from build123d import *

# Parameters (mm, degrees)
F0_W        = 186.2502396107
F0_H        = 130.5641233921
F1_DEPTH    = 50
F2_R        = 33.843412588
F3_DEPTH    = 153
F5_DEPTH    = 98
F6_T        = -2.5
F7_DEPTH    = 34.7
F8_T1_DEPTH = 77.2897189396
F8_T3_DEPTH = 80.4969668156
F8_T5_DEPTH = 71.5460241694


# Not quite as in the source:
# - a fillet or chamfer that OpenCascade refuses, or shapes differently, is made with other operations: its cross-section is extruded or revolved along the edge and cut away or added


with BuildPart() as f1:
    # F0 (on Top) → F1 (new body)
    with BuildSketch(Plane.XY):
        with Locations((-4.4038519263, -2.9969513416)):
            Rectangle(F0_W, F0_H)
    extrude(amount=F1_DEPTH)

    # F2 (on face) → F3 (cut)
    with BuildSketch(Plane(origin=(0, 0, 0), x_dir=(1, 0, 0), z_dir=(0, 0, -1))):
        with Locations((-44.7623804212, 0)):
            Circle(F2_R)
    extrude(amount=-F3_DEPTH, mode=Mode.SUBTRACT)

    # F4 (on face) → F5 (cut)
    with BuildSketch(Plane.XY.offset(50)):
        with BuildLine():
            Line((88.721267879, 62.2851103544), (43.5578748584, 62.2851103544))
            ThreePointArc((43.5578748584, 62.2851103544), (52.9449353899, 20.5157751148), (88.721267879, -2.9969513416))
            Line((88.721267879, -2.9969513416), (88.721267879, 62.2851103544))
        make_face()
    extrude(amount=-F5_DEPTH, mode=Mode.SUBTRACT)

    # F6
    f6_openings = [f1.faces().sort_by_distance(p)[0] for p in [
        (-26.985548, 62.28511, 25),
    ]]
    offset(amount=F6_T, openings=f6_openings)

    # F7 (add): a face of the model
    f7_faces = [f1.faces().sort_by_distance(p)[0] for p in [
        (-5.8734353471, -8.457374128, 50),
    ]]
    extrude(f7_faces, amount=-F7_DEPTH)

    # F8: fillet of radius 5.4579437879 on 5 edges, made by hand

    # F8_s2 → F8_t1 (cut)
    with BuildSketch(Plane.XY.offset(-13.6448594698)):
        with BuildLine():
            ThreePointArc((-97.5289717317, -62.8210692498), (-95.9303770075, -66.6804183135), (-92.0710279438, -68.2790130377))
            Line((-92.0710279438, -68.2790130377), (-97.5289717317, -68.2790130377))
            Line((-97.5289717317, -68.2790130377), (-97.5289717317, -62.8210692498))
        make_face()
        with BuildLine():
            ThreePointArc((83.2633240911, -68.2790130377), (87.1226731549, -66.6804183135), (88.721267879, -62.8210692498))
            Line((88.721267879, -62.8210692498), (88.721267879, -68.2790130377))
            Line((88.721267879, -68.2790130377), (83.2633240911, -68.2790130377))
        make_face()
        with BuildLine():
            ThreePointArc((-92.0710279438, 62.2851103544), (-95.9303770075, 60.6865156303), (-97.5289717317, 56.8271665665))
            Line((-97.5289717317, 56.8271665665), (-97.5289717317, 62.2851103544))
            Line((-97.5289717317, 62.2851103544), (-92.0710279438, 62.2851103544))
        make_face()
    extrude(amount=F8_T1_DEPTH, mode=Mode.SUBTRACT)

    # F8_s4 → F8_t3 (cut)
    with BuildSketch(Plane.XY.offset(-15.2484834078)):
        with BuildLine():
            ThreePointArc((37.4584814953, 62.2851103544), (41.4337624229, 60.5669916879), (42.9062677149, 56.4943367342))
            ThreePointArc((42.9062677149, 56.4943367342), (43.1581721547, 59.3980390485), (43.5578748584, 62.2851103544))
            Line((43.5578748584, 62.2851103544), (37.4584814953, 62.2851103544))
        make_face()
    extrude(amount=F8_T3_DEPTH, mode=Mode.SUBTRACT)

    # F8_s6 → F8_t5 (cut)
    with BuildSketch(Plane.XY.offset(-10.7730120847)):
        with BuildLine():
            ThreePointArc((88.721267879, -7.3061561755), (87.605956573, -3.99999624), (84.7158424133, -2.0450402373))
            ThreePointArc((84.7158424133, -2.0450402373), (86.7099755288, -2.557096868), (88.721267879, -2.9969513416))
            Line((88.721267879, -2.9969513416), (88.721267879, -7.3061561755))
        make_face()
    extrude(amount=F8_T5_DEPTH, mode=Mode.SUBTRACT)


solid = f1.part
The listing builds one solid part. Answer for the finished solid, in the listing's coordinates (mm). A direction names the side the tool comes from. Give positions to 0.01 mm unless a question says otherwise; leave off trailing zeros. Loops run counter-clockwise (first coordinate to the right, second up) from the corner with the lowest first, then second, coordinate; pieces in that order, holes last. Notation, with made-up numbers: (26, 35) - (82, 35) arc R26 cw to (82, 74) - close; hole circle Ø7 at (32, 85). An arc over 180 degrees is marked (long way). Answer as a JSON object with one key per item and string values.
1. A cutting plane is placed at A-A (y = -22.5). Write down the section's boundary in (x, z).
Determined:
{"outline": "(-97.53, 0) - (-70.04, 0) - (-70.04, 50) - (-97.53, 50) - close; (-19.48, 0) - (88.72, 0) - (88.72, 50) - (-19.48, 50) - close; hole (-95.03, 2.5) - (-73.3, 2.5) - (-73.3, 15.3) - (-95.03, 15.3) - close; hole (-16.22, 2.5) - (86.22, 2.5) - (86.22, 15.3) - (-16.22, 15.3) - close"}
2. Find the intervals of material crossed by L1, parallel to Z at x = 14.5, y = 32; L2, parallel to Y at x = -57, z = 3; L3, parallel to X at y = 22, z = 8, in increasing order. Write a range as [from, to].
Determined:
{"L1": "[0, 2.5], [15.3, 50]", "L2": "[-68.28, -65.78], [-34.22, -31.55], [31.55, 34.22]", "L3": "[-97.53, -95.03], [-73.69, -70.48], [-19.05, -15.83], [49, 51.95]"}
3. For faces 4 (the flat face through (-95.029, -3, 9)), 5 (the cylindrical face through (87.08, -66.72, 24.65)), 6 (the flat face through (-6, -65.779, 9)), determine the directions among +Z, -Z, +X, -X, +Y, -Y from which every point of the face is accessible in a straight line to the end or side of a thin tool.
Determined:
{"face 4": "+Y", "face 5": "+Z, -Z, +X, -Y", "face 6": "none"}
4. A cutting plane is placed at D-D (z = 9.5). Write down the section's boundary in (x, y).
Determined:
{"outline": "(-97.53, -62.82) arc R5.46 ccw to (-92.07, -68.28) - (83.26, -68.28) arc R5.46 ccw to (88.72, -62.82) - (88.72, -7.31) arc R5.46 ccw to (84.72, -2.05) arc R57.12 cw to (42.91, 56.49) arc R5.46 ccw to (40.85, 61.1) arc R59.62 ccw to (86.22, -5.01) - (86.22, -65.78) - (-95.03, -65.78) - (-95.03, 61.41) arc R5.46 ccw to (-97.53, 56.83) - close; circle Ø72.69 at (-44.76, 0); hole circle Ø67.69 at (-44.76, 0)"}
5. A cutting plane is placed at C-C (y = -43.5). Write down the section's boundary in (x, z).
Determined:
{"outline": "(-97.53, 0) - (88.72, 0) - (88.72, 50) - (-97.53, 50) - close; hole (-95.03, 2.5) - (86.22, 2.5) - (86.22, 15.3) - (-95.03, 15.3) - close"}
6. For a pull along Y with two mould halves and no side action, classify faces 1 (the flat face through (88.721, -35, 25)), 2 (the flat face through (-28, 62.285, 32)), 3 (the cylindrical face through (-10.1, -10.92, 8.81)) as pulls with the +Y half, pulls with the -Y half, needs draft (parallel to the pull), parting line crosses it, or undercut.
Determined:
{"face 1": "needs draft", "face 2": "pulls with the +Y half", "face 3": "undercut"}
7. A cutting plane is placed at B-B (x = -32.5). Write down the section's boundary in (y, z), then the cut area to 3 significant figures.
Determined:
{"outline": "(-68.28, 0) - (-31.54, 0) - (-31.54, 50) - (-68.28, 50) - close; (31.54, 0) - (62.29, 0) - (62.29, 2.5) - (34.21, 2.5) - (34.21, 15.3) - (62.29, 15.3) - (62.29, 50) - (31.54, 50) - close; hole (-65.78, 2.5) - (-34.21, 2.5) - (-34.21, 15.3) - (-65.78, 15.3) - close", "area": "2,610 mm²"}
8. Flat-ended cylindrical pins translate along their axes: pin 1 Ø1 at (y, z) = (44.5, 25) entering from +X; pin 2 Ø3 at (x, z) = (66.5, 14.5) entering from +Y; pin 3 Ø2 at (y, z) = (-1.5, 6) entering from +X. Find the tip coordinate at first contact, or state that the pin passes through.
Determined:
{"pin 1": "x = 43.52", "pin 2": "y = 7.81", "pin 3": "x = 85.85"}
